```python
from build123d import *

# Parameters (mm, degrees)
F0_R     = 14.121323
F1_DEPTH = 7
F0_W     = 2
F0_H     = 50.568709
F2_DEPTH = 42


with BuildPart() as f1:
    # F0 (on Front) → F1 (new body)
    with BuildSketch(Plane.XZ):
        Polygon((25.4, 25.4), (-25.4, 25.4), (-25.4, -25.4), (25.4, -25.4), (25.4, 25.168709), align=None)
        Circle(F0_R, mode=Mode.SUBTRACT)
    extrude(amount=F1_DEPTH)

    # F0 (on Front) → F2 (join)
    with BuildSketch(Plane.XZ):
        Polygon((25.4, 25.4), (-25.4, 25.4), (-25.4, -25.4), (25.4, -25.4), (25.4, 25.168709), align=None)
        Circle(F0_R, mode=Mode.SUBTRACT)
        with Locations((26.4, -0.115645)):
            Rectangle(F0_W, F0_H)
    extrude(amount=F2_DEPTH)


solid = f1.part
```
The listing builds one solid part. Answer for the finished solid, in the listing's coordinates (mm). A direction names the side the tool comes from. Coordinates: 2 decimals unless noted, no trailing zeros. Write each loop counter-clockwise with the first axis right and the second up, starting at its lowest first coordinate (ties: lowest second). Pieces come first, ordered by that corner, then holes. Notation, with made-up numbers: (39.25, 43) - (82.25, 43) arc R33 ccw to (82.25, 80) - close; hole circle Ø10 at (82, 11). An arc over 180 degrees is marked (long way). One line per item, written item: value.
1) A tool of negligible diameter and unlimited length cuts with its end or side. For faces 1 (the flat face through (27.4, -21, 0)), 2 (the flat face through (26, -21, 25.169)), from which of +Z, -Z, +X, -X, +Y, -Y can it reach the whole face along a straight path? Write none if from no direction.
Geometry check:
face 1: +Z, -Z, +X, +Y, -Y
face 2: +Z, +X, +Y, -Y
2) Find section B-B (y = -24.5). Give the vertices of the cut face in (x, z).
Geometry check:
outline: (-25.4, -25.4) - (27.4, -25.4) - (27.4, 25.17) - (25.4, 25.17) - (25.4, 25.4) - (-25.4, 25.4) - close; hole circle Ø28.24 at (0, 0)
3) Find section A-A (x = 0). Give the vertices of the cut face in (y, z), and give its area (3 significant figures).
Geometry check:
outline: (-42, -25.4) - (0, -25.4) - (0, -14.12) - (-42, -14.12) - close; (-42, 14.12) - (0, 14.12) - (0, 25.4) - (-42, 25.4) - close
area: 947 mm2
4) This flat-tipped pin is pushed along its axis until it touches: pin 1 Ø0.6 at (x, y) = (27, -13.5) entering from +Z. Where does it stop, or does it pass through?
Geometry check:
pin 1: stops at z = 25.17
5) For a pull along X with two mould halves and no side action, classify faces 3 (the flat face through (-25.4, -21, 0)), 4 (the cylindrical face through (-11.2, -20.7, -8.6)), 5 (the flat face through (-11, 0, -11)) as pulls with the +X half, pulls with the -X half, needs draft (parallel to the pull), parting line crosses it, or undercut.
Geometry check:
face 3: pulls with the -X half
face 4: undercut
face 5: needs draft
6) Consider line 1 along Z through (x, y) = (0, -14.5); line 2 along X through (y, z) = (-9.5, 0.5); line 3 along X through (y, z) = (-15.5, 8). Determine where each line is inside the solid, lowest interval first. Write a range as from..to.
Geometry check:
line 1: z = -25.4..-14.12, 14.12..25.4
line 2: x = -25.4..-14.11, 14.11..27.4
line 3: x = -25.4..-11.64, 11.64..27.4
7) Find section C-C (z = 0). Give the vertices of the cut face in (x, y).
Geometry check:
outline: (-25.4, -42) - (-14.12, -42) - (-14.12, 0) - (-25.4, 0) - close; (14.12, -42) - (27.4, -42) - (27.4, 0) - (14.12, 0) - close
